from build123d import *

# Parameters (mm, degrees)
F0_R     = 14.2875
F1_DEPTH = 9.525
F2_R     = 5.08


with BuildPart() as f1:
    # F0 (on Front) → F1 (new body, symmetric)
    with BuildSketch(Plane.XZ):
        with BuildLine():
            ThreePointArc((317.5, 146.05), (280.478203, 107.965259), (241.361025, 143.894458))
            ThreePointArc((241.361025, 143.894458), (235.097549, 154.13599), (223.100917, 154.584212))
            ThreePointArc((223.100917, 154.584212), (196.448532, 144.511932), (168.387104, 139.576686))
            ThreePointArc((168.387104, 139.576686), (150.974575, 133.730468), (138.320821, 120.416681))
            Line((138.320821, 120.416681), (82.55, 22.225))
            ThreePointArc((82.55, 22.225), (156.404838, 50.655649), (234.95, 60.325))
            Line((234.95, 60.325), (400.05, 60.325))
            Line((400.05, 60.325), (400.05, 9.525))
            Line((400.05, 9.525), (412.75, 9.525))
            ThreePointArc((412.75, 9.525), (452.222526, 73.519998), (501.65, 130.18008))
            Line((501.65, 130.18008), (449.9643, 127.06884))
            ThreePointArc((449.9643, 127.06884), (409.702523, 161.985365), (443.736498, 202.995886))
            Line((443.736498, 202.995886), (476.25, 206.375))
            ThreePointArc((476.25, 206.375), (448.550685, 233.798385), (409.575, 233.3625))
            Line((409.575, 233.3625), (317.5, 193.675))
            Line((317.5, 193.675), (317.5, 146.05))
        make_face()
        with Locations((171.45, 101.6)):
            Circle(F0_R, mode=Mode.SUBTRACT)
    extrude(amount=F1_DEPTH, both=True)

    # F2
    f2_edges = [f1.edges().sort_by_distance(p)[0] for p in [
        (317.5, 0, 193.675),
        (476.25, 0, 206.375),
        (501.65, 0, 130.18008),
        (412.75, 0, 9.525),
        (400.05, 0, 60.325),
    ]]
    fillet(f2_edges, radius=F2_R)


solid = f1.part
Geometry: final body of the model. Coordinates: model frame, mm. A direction names the side the tool comes from. Give positions to 0.01 mm unless a question says otherwise; leave off trailing zeros. Write each loop counter-clockwise with the first axis right and the second up, starting at its lowest first coordinate (ties: lowest second). Pieces come first, ordered by that corner, then holes.
(1) Mould query, pull axis Z, two halves, no side actions, for faces 5 (the flat face through (400.05, 0, 33)), 6 (the flat face through (110.826, -0.133, 72.008)), 7 (the flat face through (456.143, -0.133, 204.285)), 8 (the cylindrical face through (184.65, 0.13, 96.13)). Classes: released by +Z, released by -Z, zero draft, split by the parting line, or undercut.
(2) Ray query, line 1 (X direction, y = 1, z = 134); line 2 (Z direction, x = 171.45, y = 1.75); line 3 (Z direction, x = 171, y = -2). Return the intervals inside material, ascending.
(3) Cut plane C-C, the plane z = 101.6. Return loops of the section in (x, y) (1 decimal).
(4) Cut plane D-D, the plane x = 279.4. Return loops of the section in (y, z) (3 decimals).
(5) Cut plane B-B, the plane x = 421. Return loops of the section in (y, z) (3 decimals).
(6) Access query for faces 1 (the flat face through (314, 0, 60.325)), 2 (the cylindrical face through (151.194, -0.133, 133.869)), 3 (the flat face through (317.5, 0, 169)), 4 (the flat face through (469.4, -0.13, 128.24)). Directions: +Z, -Z, +X, -X, +Y, -Y. A direction counts if a zero-diameter tool reaches every point of the face in a straight line with its end or side. Return the directions, or none.
(7) First-contact query: P1, Ø9.5, axis at y = 1.5, z = 172.5, coming from the -X side; P2, Ø9.5, axis at y = -4, z = 40, coming from the -X side; P3, Ø9.5, axis at x = 307, y = 3.5, coming from the -Z side (3 decimals). Flat tips, straight axial feed; report the tip coordinate or a pass-through.
Values follow:
1. face 5: zero draft
1. face 6: released by +Z
1. face 7: undercut
1. face 8: undercut
2. line 1: x = 151.4 to 243.26, 315.54 to 425.67
2. line 2: z = 54.04 to 87.31, 115.89 to 139.85
2. line 3: z = 53.95 to 87.32, 115.88 to 139.81
3. outline: (127.6, -9.5) - (157.2, -9.5) - (157.2, 9.5) - (127.6, 9.5) - close; (185.7, -9.5) - (474.7, -9.5) - (474.7, 9.5) - (185.7, 9.5) - close
4. outline: (-9.525, 60.325) - (9.525, 60.325) - (9.525, 107.95) - (-9.525, 107.95) - close
5. outline: (-9.525, 25.009) - (9.525, 25.009) - (9.525, 137.896) - (-9.525, 137.896) - close; (-9.525, 192.304) - (9.525, 192.304) - (9.525, 236.757) - (-9.525, 236.757) - close
6. face 1: -Z, +Y, -Y
6. face 2: +Z, -X, +Y, -Y
6. face 3: +Z, +Y, -Y
6. face 4: +Y, -Y
7. P1: stops at x = 317.5
7. P2: stops at x = 89.95
7. P3: stops at z = 60.325
